Could you check a few things on this model? Use its own coordinates, in mm. Face numbers are marked on the shaded views. A direction names the side the tool comes from. Round coordinates to 2 decimals unless told otherwise and drop trailing zeros. Write each loop counter-clockwise with the first axis right and the second up, starting at its lowest first coordinate (ties: lowest second). Pieces come first, ordered by that corner, then holes. Notation, with made-up numbers: (-16, 4.5) - (21, 4.5) arc R29 cw to (21, 25.5) - close; hole circle Ø11 at (47.25, 85.25). An arc over 180 degrees is marked (long way). Write each question's results on one line, items separated by ' | '. Start each with the question number.
(1) For P1, Ø5, axis at x = 1, z = 6.5, coming from the +Y side; P2, Ø6, axis at x = -1.5, z = 13, coming from the +Y side, each with a flat end and sliding along its axis, tell me the tip position at first contact or that it passes through.
(2) Imagine slicing it at D-D on x = -15. Write out the boundary of the cut face in (y, z) (3 decimals).
(3) Imagine slicing it at A-A on x = 15. Write out the boundary of the cut face in (y, z) (3 decimals).
(4) On a 3-axis mill with a long thin cutter (end or side, diameter ignored), from which of +Z, -Z, +X, -X, +Y, -Y can I reach the whole of each face in a straight line? I mean the marked faces 1, 2, 3, 4 and 5. Say none if no direction works.
(5) Please list where these lines run through material, in increasing order: line 1 (Z direction, x = 15, y = 10); line 2 (Z direction, x = -15, y = 6.5); line 3 (X direction, y = -1.5, z = 1). Write a range as [from, to].
(6) Thinking about a two-plate mould opening in X: for the marked faces 6, 7 and 8, which applies, +X half, -X half, draft (parallel to the pull), parting line (faces both ways), or undercut?
(7) Imagine slicing it at C-C on z = 3.5. Write out the boundary of the cut face in (x, y) (3 decimals).
(8) Imagine slicing it at B-B on y = 3. Write out the boundary of the cut face in (x, z) (3 decimals).
```python
from build123d import *

# Parameters (mm, degrees)
F1_DEPTH = 14.5
F2_W     = 12.5
F2_H     = 14.5
F3_DEPTH = 0.1
F4_W     = 2
F4_H     = 3.5
F4_W_2   = 25.25
F5_DEPTH = 4.175
F6_W     = 2
F6_H     = 3.6
F6_W_2   = 25.25
F7_DEPTH = 4.175
F8_W     = 27.65
F8_H     = 3.5
F9_DEPTH = 4.175


with BuildPart() as f1:
    # F0 (on Top) → F1 (new body)
    with BuildSketch(Plane.XY):
        with BuildLine():
            Line((-18, 11.625), (-18, -13.625))
            Line((-18, -13.625), (18, -13.625))
            Line((18, -13.625), (18, 11.625))
            ThreePointArc((18, 11.625), (17.4142135624, 13.0392135624), (16, 13.625))
            Line((16, 13.625), (-16, 13.625))
            ThreePointArc((-16, 13.625), (-17.4142135624, 13.0392135624), (-18, 11.625))
        make_face()
        with BuildLine():
            ThreePointArc((5.8984604593, -1.8097746648), (0, -7.575), (-5.8984604593, -1.8097746648))
            Line((-5.8984604593, -1.8097746648), (-6.25, 13.5754765943))
            Line((-6.25, 13.5754765943), (6.25, 13.5754765943))
            Line((6.25, 13.5754765943), (5.8984604593, -1.8097746648))
        make_face(mode=Mode.SUBTRACT)
    extrude(amount=F1_DEPTH)

    # F2 (on face) → F3 (cut)
    with BuildSketch(Plane(origin=(0, 13.625, 0), x_dir=(-1, 0, 0), z_dir=(0, 1, 0))):
        with Locations((-0.0153454952, 7.25)):
            Rectangle(F2_W, F2_H)
    extrude(amount=-F3_DEPTH, mode=Mode.SUBTRACT)

    # F4 (on face) → F5 (cut)
    with BuildSketch(Plane.YZ.offset(18)):
        with Locations((12.625, 11.25)):
            Rectangle(F4_W, F4_H)
        with Locations((-1, 11.25)):
            Rectangle(F4_W_2, F4_H)
    extrude(amount=-F5_DEPTH, mode=Mode.SUBTRACT)

    # F6 (on face) → F7 (cut)
    with BuildSketch(Plane(origin=(-18, 0, 0), x_dir=(0, -1, 0), z_dir=(-1, 0, 0))):
        with Locations((-12.625, 11.2)):
            Rectangle(F6_W, F6_H)
        with Locations((1, 11.2)):
            Rectangle(F6_W_2, F6_H)
    extrude(amount=-F7_DEPTH, mode=Mode.SUBTRACT)

    # F8 (on face) → F9 (cut)
    with BuildSketch(Plane.XZ.offset(13.625)):
        with Locations((0, 11.25)):
            Rectangle(F8_W, F8_H)
    extrude(amount=-F9_DEPTH, mode=Mode.SUBTRACT)


solid = f1.part
```
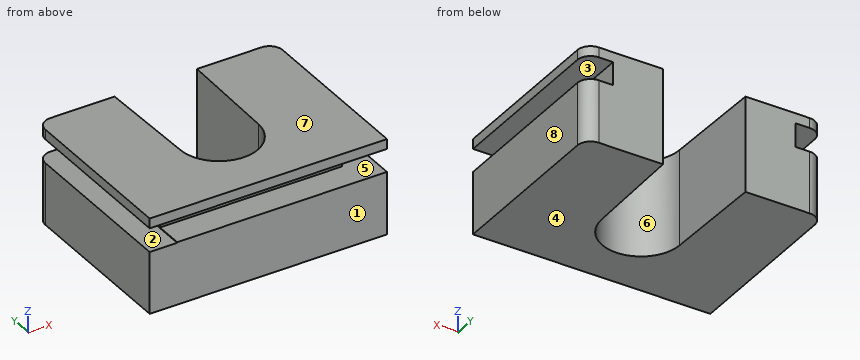
Response:
1) P1: y = -6.42 | P2: y = -5.49
2) outline: (-13.625, 0) - (13.625, 0) - (13.625, 9.4) - (-13.625, 9.4) - close; (-13.625, 13) - (13.625, 13) - (13.625, 14.5) - (-13.625, 14.5) - close
3) outline: (-13.625, 0) - (13.625, 0) - (13.625, 9.5) - (-13.625, 9.5) - close; (-13.625, 13) - (13.625, 13) - (13.625, 14.5) - (-13.625, 14.5) - close
4) face 1: +Z, -Z, +X, -X, -Y | face 2: -X, +Y, -Y | face 3: -Y | face 4: -Z, +X, -X, +Y, -Y | face 5: +X, -Y
5) line 1: [0, 9.5], [13, 14.5] | line 2: [0, 9.4], [13, 14.5] | line 3: [-18, -5.91], [5.91, 18]
6) face 6: undercut | face 7: draft | face 8: +X half
7) outline: (-18, -13.625) - (18, -13.625) - (18, 11.625) arc R2 ccw to (16, 13.625) - (6.265, 13.625) - (6.265, 13.525) - (6.249, 13.525) - (5.898, -1.81) arc R5.9 cw to (-5.898, -1.81) - (-6.25, 13.575) - (-6.235, 13.575) - (-6.235, 13.625) - (-16, 13.625) arc R2 ccw to (-18, 11.625) - close
8) outline: (-18, 0) - (-6.008, 0) - (-6.008, 14.5) - (-18, 14.5) - (-18, 13) - (-13.825, 13) - (-13.825, 9.4) - (-18, 9.4) - close; (6.008, 0) - (18, 0) - (18, 9.5) - (13.825, 9.5) - (13.825, 13) - (18, 13) - (18, 14.5) - (6.008, 14.5) - close
